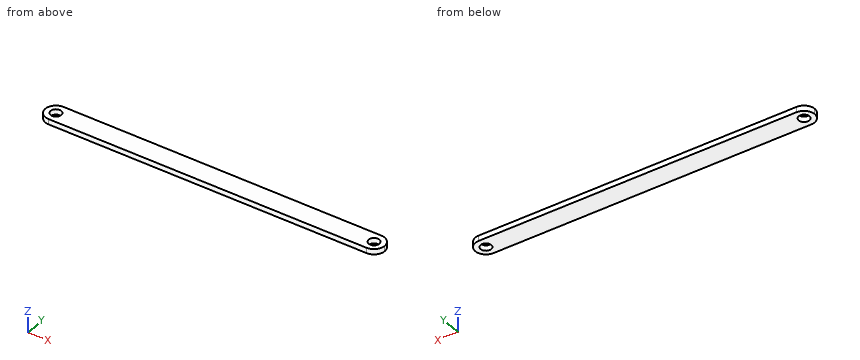
Solid Edge part; units mm, degrees
sketch "Sketch1" plane through (0, 0, 0) normal (0, 0, 1) x (1, 0, 0)
  line L0 (160, -10) -> (-160, -10)
  line L1 (-160, -10) -> (-160, 10)
  line L2 (-160, 10) -> (160, 10)
  line L3 (160, 10) -> (160, -10)
  circle A0 centre (-150, 0) radius 5
  circle A1 centre (150, 0) radius 5
  dimension "D1" = 160
  dimension "D2" = 160
extrude "Protrusion1" add sketch "Sketch1" along normal blind 5
fillet "Round_1" radius 10 4 edges at (160, -10, 2.5) (160, 10, 2.5) (-160, 10, 2.5) (-160, -10, 2.5)
Read the model definition and answer for the solid it produces. Units are mm, in the model's axes. Give positions to 0.01 mm unless a question says otherwise; leave off trailing zeros. Answer as a JSON object with one key per item and string values. Group by question number.
1) Each of these flat-tipped pins is pushed along its axis until it touches: P1, Ø6, axis at x = 50, y = -4, coming from the -Z side; P2, Ø1.5, axis at y = 4.5, z = 3, coming from the -X side; P3, Ø2, axis at y = 3, z = 0.5, coming from the -X side; P4, Ø8, axis at x = -150, y = 0, coming from the -Z side. Where does it stop, or does it pass through?
2) Consider L1, parallel to X at y = 0.5, z = 3.25; L2, parallel to X at y = -3.25, z = 4.65; L3, parallel to Y at x = -150, z = 3.7. Determine where each line is inside the solid, lowest interval first. Write a range as from..to.
3) Find section A-A (z = 1.7). Count the separate pieces of the cut face and the enclosed holes in it, and give its area (3 significant figures).
Values follow:
{
 "1": {"P1": "stops at z = 0", "P2": "stops at x = -159.27", "P3": "stops at x = -159.8", "P4": "passes through"},
 "2": {"L1": "x = -159.99..-154.97, -145.03..145.03, 154.97..159.99", "L2": "x = -159.46..-153.8, -146.2..146.2, 153.8..159.46", "L3": "y = -10..-5, 5..10"},
 "3": {"separate pieces": "1", "enclosed holes": "2", "area": "6,160 mm2"}
}
